```python
from build123d import *

# Parameters (mm, degrees)
F0_R     = 10
F1_DEPTH = 8


with BuildPart() as f1:
    # F0 (on Top) → F1 (new body)
    with BuildSketch(Plane.XY):
        with BuildLine():
            ThreePointArc((-69.624749, 4.596739), (-40.217301, -2.204414), (-14.178766, -17.470335))
            ThreePointArc((-14.178766, -17.470335), (20.016237, -10.276199), (5.932914, 21.703698))
            ThreePointArc((5.932914, 21.703698), (-33.628428, 28.347466), (-73.71984, 26.962516))
            ThreePointArc((-73.71984, 26.962516), (-89.508922, 19.750139), (-98.660254, 5))
            Line((-98.660254, 5), (-100, 0))
            Line((-100, 0), (-104.019238, -15))
            Line((-104.019238, -15), (-103.242781, -17.897777))
            ThreePointArc((-103.242781, -17.897777), (-90.392251, -17.560317), (-79.094635, -11.427301))
            Line((-79.094635, -11.427301), (-79.871092, -8.529524))
            ThreePointArc((-79.871092, -8.529524), (-78.264558, 0.77869), (-69.624749, 4.596739))
        make_face()
        Circle(F0_R, mode=Mode.SUBTRACT)
        with BuildLine():
            ThreePointArc((-16.033026, 18.300115), (-12.916015, 15.72181), (-13.642437, 11.742398))
            ThreePointArc((-13.642437, 11.742398), (-16.529122, 7.12658), (-17.903763, 1.858839))
            ThreePointArc((-17.903763, 1.858839), (-20.05158, -1.284513), (-23.857845, -1.206234))
            ThreePointArc((-23.857845, -1.206234), (-45.676184, 8.182002), (-69.019088, 12.57378))
            ThreePointArc((-69.019088, 12.57378), (-78.904215, 10.480055), (-86.103752, 3.390197))
            ThreePointArc((-86.103752, 3.390197), (-89.022149, 2.455102), (-90.149125, 5.304904))
            ThreePointArc((-90.149125, 5.304904), (-83.259717, 14.546079), (-72.643211, 19.035293))
            ThreePointArc((-72.643211, 19.035293), (-44.310872, 20.765745), (-16.033026, 18.300115))
        make_face(mode=Mode.SUBTRACT)
    extrude(amount=-F1_DEPTH)


solid = f1.part
```
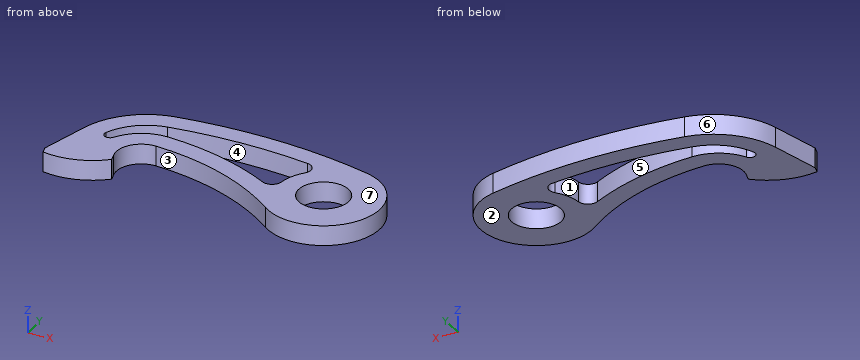
Geometry: final body of the model. Coordinates: model frame, mm. Face numbers are marked on the shaded views. A direction names the side the tool comes from. Round coordinates to 2 decimals unless told otherwise and drop trailing zeros. Write each loop counter-clockwise with the first axis right and the second up, starting at its lowest first coordinate (ties: lowest second). Pieces come first, ordered by that corner, then holes.
Item 1: Section query B-B (y = -3.5). Return loops of the section in (x, z), plus the area to 3 significant figures.
Item 2: Mould query, pull axis Y, two halves, no side actions, for the marked faces 4, 5, 6 and 7. Classes: +Y half, -Y half, draft (parallel to the pull), parting line (faces both ways), or undercut.
Item 3: Section query A-A (z = -3.5). Return loops of the section in (x, y).
Item 4: Section query C-C (x = -48.5). Return loops of the section in (y, z).
Item 5: Pin query (flat end, axial travel): P1, Ø1.5, axis at x = -13, z = -1.5, coming from the +Y side; P2, Ø3, axis at x = -76.5, z = -4.5, coming from the +Y side; P3, Ø10, axis at x = -39, y = 6.5, coming from the -Z side; P4, Ø1.5, axis at y = 4, z = -2.5, coming from the -X side. Return the tip coordinate at first contact, or that it passes through.
Item 6: Set-up query: the marked faces 1, 2 and 3. Return all of +Z, -Z, +X, -X, +Y, -Y with unobstructed straight access to the full face (end or side cutting, diameter ignored); none if empty.
Item 7: Section query D-D (x = 0). Return loops of the section in (y, z).
Item 8: Material intervals for L1, parallel to Y at x = -18.5, z = -7; L2, parallel to Y at x = 0, z = -6.25; L3, parallel to X at y = 14, z = -7, sorted ascending.
Completed:
1. outline: (-100.94, -8) - (-80.2, -8) - (-80.2, 0) - (-100.94, 0) - close; (-37.11, -8) - (-9.37, -8) - (-9.37, 0) - (-37.11, 0) - close; (9.37, -8) - (22.23, -8) - (22.23, 0) - (9.37, 0) - close
1. area: 491 mm2
2. face 4: undercut
2. face 5: undercut
2. face 6: +Y half
2. face 7: draft
3. outline: (-104.02, -15) - (-103.24, -17.9) arc R27.54 ccw to (-79.09, -11.43) - (-79.87, -8.53) arc R10 cw to (-69.62, 4.6) arc R100 cw to (-14.18, -17.47) arc R22.5 ccw (long way) to (5.93, 21.7) arc R200 ccw to (-73.72, 26.96) arc R30 ccw to (-98.66, 5) - close; hole (-90.15, 5.3) arc R2.24 ccw to (-86.1, 3.39) arc R18 cw to (-69.02, 12.57) arc R108 cw to (-23.86, -1.21) arc R4 ccw to (-17.9, 1.86) arc R18 cw to (-13.64, 11.74) arc R4 ccw to (-16.03, 18.3) arc R192 ccw to (-72.64, 19.04) arc R22 ccw to start; hole circle Ø20 at (0, 0)
4. outline: (0.68, -8) - (9, -8) - (9, 0) - (0.68, 0) - close; (20.77, -8) - (28.77, -8) - (28.77, 0) - (20.77, 0) - close
5. P1: stops at y = 26.03
5. P2: stops at y = 26.76
5. P3: stops at z = -8
5. P4: stops at x = -99.13
6. face 1: +Z, -Z
6. face 2: -Z, +X, -X, +Y, -Y
6. face 3: +Z, -Z, -Y
7. outline: (-22.5, -8) - (-10, -8) - (-10, 0) - (-22.5, 0) - close; (10, -8) - (23.23, -8) - (23.23, 0) - (10, 0) - close
8. L1: y = -14.15 to 0.14, 18.68 to 26.77
8. L2: y = -22.5 to -10, 10 to 23.23
8. L3: x = -94.56 to -83.93, -12.69 to 17.61
